Design review of the part built by this model. Coordinates are the model's own, in mm. A direction names the side the tool comes from. Give positions to 0.01 mm unless a question says otherwise; leave off trailing zeros. Order: outer loops, then holes, each group sorted by start corner. A loop starts at its lowest first (then second) coordinate and runs counter-clockwise, first axis right, second up. Notation, with made-up numbers: (78, 6.5) -> (82, 6.5) arc R35 ccw to (82, 42.5) -> close; hole circle Ø11 at (44.25, 69.25). An arc over 180 degrees is marked (long way). Answer in a Markdown table with one row per item. Add a question column.
```python
from build123d import *

# Parameters (mm, degrees)
CYLINDER006_R     = 26.7
CYLINDER006_DEPTH = 7.25
CYLINDER007_R     = 4.5
CYLINDER007_DEPTH = 32
CYLINDER005_R     = 26.7
CYLINDER005_DEPTH = 7.25
CYLINDER004_R     = 32
CYLINDER004_DEPTH = 6.5


with BuildPart() as cylinder006:
    # Cylinder006 → Cylinder006 (new body)
    with BuildSketch(Plane.XY.offset(7.75)):
        Circle(CYLINDER006_R)
    extrude(amount=CYLINDER006_DEPTH)


with BuildPart() as cylinder007:
    # Cylinder007 → Cylinder007 (new body)
    with BuildSketch(Plane.XY):
        Circle(CYLINDER007_R)
    extrude(amount=CYLINDER007_DEPTH)


with BuildPart() as fusion003:
    # Cylinder005 → Cylinder005 (new body)
    with BuildSketch(Plane.XY.offset(17)):
        Circle(CYLINDER005_R)
    extrude(amount=CYLINDER005_DEPTH)

    # Fusion003: union Cylinder006, Cylinder007
    add(cylinder006.part)
    add(cylinder007.part)


with BuildPart() as cone002:
    # Cone002 → Cone002 (revolve)
    with BuildSketch(Plane(origin=(0, 0, 8.5), x_dir=(1, 0, 0), z_dir=(0, -1, 0))):
        Polygon((0, 0), (32, 0), (30, 2), (0, 2), align=None)
    revolve(axis=Axis((0, 0, 8.5), (0, 0, 1)))


with BuildPart() as cone003:
    # Cone003 → Cone003 (revolve)
    with BuildSketch(Plane.XZ):
        Polygon((0, 0), (30, 0), (32, 2), (0, 2), align=None)
    revolve(axis=Axis((0, 0, 0), (0, 0, 1)))


with BuildPart() as cut:
    # Cylinder004 → Cylinder004 (new body)
    with BuildSketch(Plane.XY.offset(2)):
        Circle(CYLINDER004_R)
    extrude(amount=CYLINDER004_DEPTH)

    # Fusion002: union Cone002, Cone003
    add(cone002.part)
    add(cone003.part)


with BuildPart() as cut_1:
    # Fusion002 placement: moved
    add(cut.part.moved(Location((0, 0, 10.75))))

    # Cut: cut Fusion003
    add(fusion003.part, mode=Mode.SUBTRACT)


solid = cut_1.part
```
1) Add section C-C, the plane z = 15.75. Write out the cut boundary in (x, y).
2) For L1, parallel to Y at x = 0, z = 15.45; L2, parallel to Y at x = 0, z = 13.25; L3, parallel to Z at x = -22.5, y = 3, list the stretches that pass through material, from the lowest coordinate up.
3) Clearance check with flat-ended pins moving along their axes: P1, Ø1.5, axis at x = -3, z = 15, coming from the -Y side; P2, Ø3, axis at x = 13, z = 15, coming from the -Y side; P3, Ø1, axis at x = -23, z = 19.5, coming from the +Y side. State where each tip first meets the part, or that it passes through.
4) Add section A-A, the plane x = 0. Write out the cut boundary in (y, z).
5) Add section D-D, the plane z = 20.25. Write out the cut boundary in (x, y).
6) Machinability: for faces 4 (the face through (-20, -18, 21.25)), 5 (the face through (25.467, 8.02, 12.845)), 6 (the face through (0, -6, 17)), which of the approach directions +Z, -Z, +X, -X, +Y, -Y give a long, thin tool a straight path to every point of the face, cutting with its end or side? Answer none if there is none.
7) Mouldability with a two-part tool opening along Y and no side actions: class faces 1 (the face through (25.467, 8.02, 19.095)), 2 (the face through (-6.531, -29.409, 10.875)), 3 (the face through (20, -18, 10.75)) as +Y half, -Y half, draft (parallel to the pull), parting line (faces both ways), or undercut.
Verdict:
| question | item | result |
|---|---|---|
| 1 | outline | circle Ø64 at (0, 0); hole circle Ø9 at (0, 0) |
| 2 | L1 | y = -32 to -4.5, 4.5 to 32 |
| 2 | L2 | y = -32 to -26.7, 26.7 to 32 |
| 2 | L3 | z = 15 to 17 |
| 3 | P1 | stops at y = -31.92 |
| 3 | P2 | stops at y = -29.86 |
| 3 | P3 | stops at y = 22.69 |
| 4 | outline | (-32, 12.75) -> (-30, 10.75) -> (-26.7, 10.75) -> (-26.7, 15) -> (-4.5, 15) -> (-4.5, 17) -> (-26.7, 17) -> (-26.7, 21.25) -> (-30, 21.25) -> (-32, 19.25) -> close; (4.5, 15) -> (26.7, 15) -> (26.7, 10.75) -> (30, 10.75) -> (32, 12.75) -> (32, 19.25) -> (30, 21.25) -> (26.7, 21.25) -> (26.7, 17) -> (4.5, 17) -> close |
| 5 | outline | circle Ø62 at (0, 0); hole circle Ø53.4 at (0, 0) |
| 6 | face 4 | +Z, +X, -X, +Y, -Y |
| 6 | face 5 | -Z |
| 6 | face 6 | +Z |
| 7 | face 1 | undercut |
| 7 | face 2 | parting line |
| 7 | face 3 | draft |
